Job drawing, mm, ordinate dimensions from the low corner. One solid piece. A direction names the side the tool comes from. Coordinates: 2 decimals unless noted, no trailing zeros. Write each loop counter-clockwise with the first axis right and the second up, starting at its lowest first coordinate (ties: lowest second). Pieces come first, ordered by that corner, then holes. Notation, with made-up numbers: M 29,46 L 58,46 A17 ccw 58,72 Z; hole C 47,72 d11. An arc over 180 degrees is marked long. Answer as CSV lines item,"result". Start each with the question number.
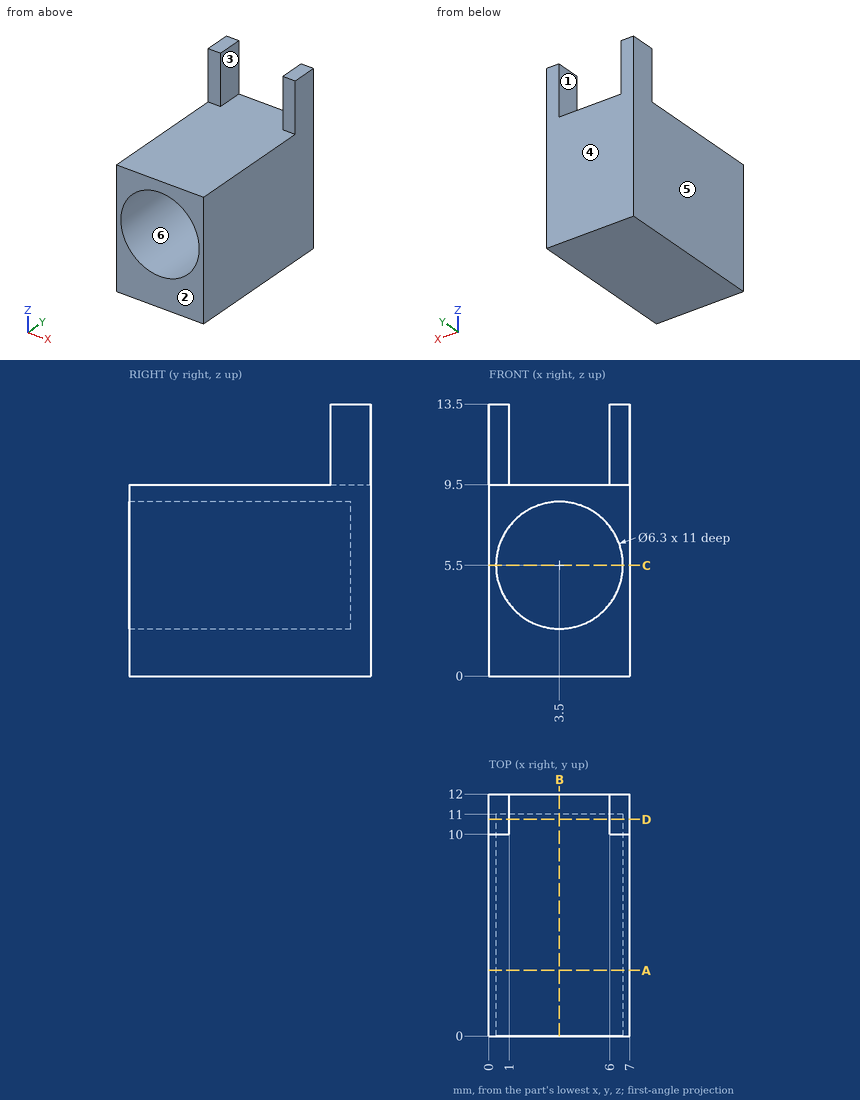
1) Band-saw the part on C-C, the plane z = 5.5. List the corners of the cut face in (x, y), plus the area to 3 significant figures.
2) Probe L1, parallel to X at y = 5, z = 5.5; L2, parallel to Y at x = 2, z = 6.75; L3, parallel to Y at x = 6.5, z = 11.25. List the from-to ranges inside material, lowest first. Write a range as [from, to].
3) Two-plate mould, pull along X, no slides. Class the marked faces 3, 4, 5 and 6: pulls with the +X half, pulls with the -X half, needs draft (parallel to the pull), parting line crosses it, or undercut.
4) Band-saw the part on D-D, the plane y = 10.75. List the corners of the cut face in (x, z), plus the area to 3 significant figures.
5) Band-saw the part on A-A, the plane y = 3.25. List the corners of the cut face in (x, z), plus the area to 3 significant figures.
6) Tool access for the marked faces 1 and 2: list every direction of +Z, -Z, +X, -X, +Y, -Y with a clear straight run to the whole face (end or side of a thin tool).
7) Pin check, flat tip, straight feed: P1, Ø0.8, axis at x = 6.5, z = 12, coming from the -Y side. Stop position of the tip, or through.
8) Band-saw the part on B-B, the plane x = 3.5. List the corners of the cut face in (y, z).
Result sheet:
1,outline,"M 0,0 L 0.35,0 L 0.35,11 L 6.65,11 L 6.65,0 L 7,0 L 7,12 L 0,12 Z"
1,area,"14.7 mm²"
2,L1,"x = [0, 0.35], [6.65, 7]"
2,L2,"y = [11, 12]"
2,L3,"y = [10, 12]"
3,face 3,"undercut"
3,face 4,"needs draft"
3,face 5,"pulls with the -X half"
3,face 6,"undercut"
4,outline,"M 0,0 L 7,0 L 7,13.5 L 6,13.5 L 6,9.5 L 1,9.5 L 1,13.5 L 0,13.5 Z; hole C 3.5,5.5 d6.3"
4,area,"43.3 mm²"
5,outline,"M 0,0 L 7,0 L 7,9.5 L 0,9.5 Z; hole C 3.5,5.5 d6.3"
5,area,"35.3 mm²"
6,face 1,"+Z, +Y, -Y"
6,face 2,"+Z, -Z, +X, -X, -Y"
7,P1,"stops at y = 10"
8,outline,"M 0,0 L 12,0 L 12,9.5 L 0,9.5 L 0,8.65 L 11,8.65 L 11,2.35 L 0,2.35 Z"
